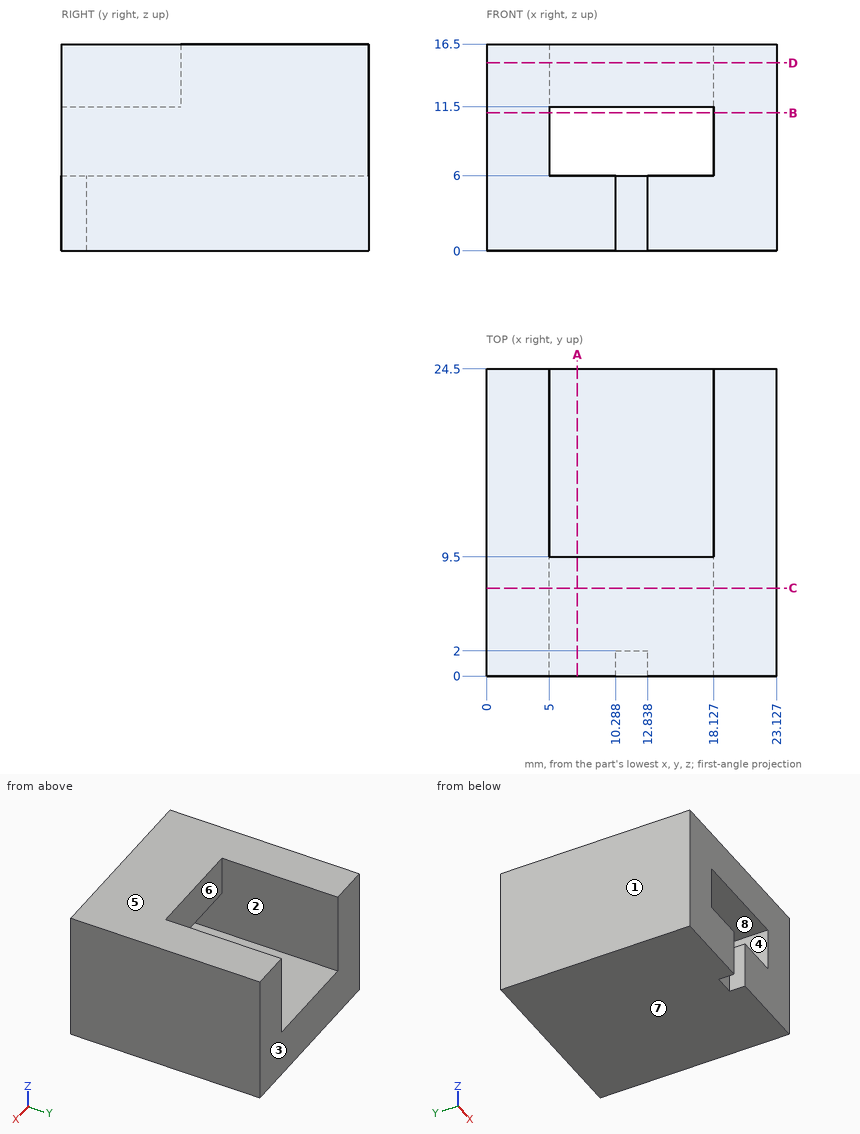
Geometry check sheet. Reference: drawing and pictorial views, mm from the part's lowest x, y, z. A direction names the side the tool comes from. Give positions to 0.01 mm unless a question says otherwise; leave off trailing zeros. Order: outer loops, then holes, each group sorted by start corner. A loop starts at its lowest first (then second) coordinate and runs counter-clockwise, first axis right, second up. Notation, with made-up numbers: M 20.25,23 L 63.25,23 A28 ccw 63.25,50 Z; hole C -17,-36 d11. An arc over 180 degrees is marked long. Answer in a Markdown table with one row per item. Add a question column.
Item 1: Tool access check on the marked faces 4, 5, 6, 7 and 8. Record the directions out of +Z, -Z, +X, -X, +Y, -Y that give a thin tool (end or side, any length) a straight path to the whole face; none if there is none.
Item 2: Section check B-B, the plane z = 11. Enter the section's corners in (x, y), and give its area (3 significant figures).
Item 3: Section check D-D, the plane z = 15. Enter the section's corners in (x, y), and give its area (3 significant figures).
Item 4: Mould release check, pull along X, two halves, no side actions. Record for the marked faces 1, 2 and 3: released by +X, released by -X, zero draft, split by the parting line, or undercut.
Item 5: Gauge pin test, flat ends, axial feed: pin 1 (5.5 mm diameter, centred on x = 11.5, z = 13.5, fed in from +Y); pin 2 (6 mm diameter, centred on x = 14, z = 13.5, fed in from -Y); pin 3 (6.5 mm diameter, centred on x = 9.5, y = 13, fed in from +Z). Record the tip position at first contact, or that the pin passes through.
Item 6: Section check A-A, the plane x = 7.25. Enter the section's corners in (y, z).
Item 7: Section check C-C, the plane y = 7. Enter the section's corners in (x, z).
Item 8: Scan lines: probe 1 along Z at (x, y) = (9, 6.25); probe 2 along X at (y, z) = (13, 13.5); probe 3 along Z at (x, y) = (12.75, 19.25). Record each from-to range of solid material in increasing order. Write a range as from..to.
Filled sheet:
| question | item | result |
|---|---|---|
| 1 | face 4 | +Y |
| 1 | face 5 | +Z, +X, -X, +Y, -Y |
| 1 | face 6 | +Z, +Y |
| 1 | face 7 | -Z, +X, -X, +Y, -Y |
| 1 | face 8 | +Y, -Y |
| 2 | outline | M 0,0 L 5,0 L 5,24.5 L 0,24.5 Z; M 18.13,0 L 23.13,0 L 23.13,24.5 L 18.13,24.5 Z |
| 2 | area | 245 mm^2 |
| 3 | outline | M 0,0 L 23.13,0 L 23.13,24.5 L 18.13,24.5 L 18.13,9.5 L 5,9.5 L 5,24.5 L 0,24.5 Z |
| 3 | area | 370 mm^2 |
| 4 | face 1 | released by -X |
| 4 | face 2 | undercut |
| 4 | face 3 | zero draft |
| 5 | pin 1 | stops at y = 9.5 |
| 5 | pin 2 | stops at y = 0 |
| 5 | pin 3 | stops at z = 6 |
| 6 | outline | M 0,0 L 24.5,0 L 24.5,6 L 0,6 Z; M 0,11.5 L 9.5,11.5 L 9.5,16.5 L 0,16.5 Z |
| 7 | outline | M 0,0 L 23.13,0 L 23.13,16.5 L 0,16.5 Z; hole M 5,6 L 18.13,6 L 18.13,11.5 L 5,11.5 Z |
| 8 | probe 1 | z = 0..6, 11.5..16.5 |
| 8 | probe 2 | x = 0..5, 18.13..23.13 |
| 8 | probe 3 | z = 0..6 |
